The model under review builds one solid part; all positions refer to its coordinate system, in mm. Face numbers are marked on the shaded views. A direction names the side the tool comes from. Give positions to 0.01 mm unless a question says otherwise; leave off trailing zeros. Loops run counter-clockwise (first coordinate to the right, second up) from the corner with the lowest first, then second, coordinate; pieces in that order, holes last. Notation, with made-up numbers: M 8.5,-1 L 30.5,-1 A13 ccw 30.5,21 Z; hole C 18.25,31.5 d10. An arc over 180 degrees is marked long. Write item = value, one per line. Start each with the question number.
1. Draft analysis for pull direction X (two halves, no side actions). For the marked faces 1, 2, 3 and 4, state which applies: pulls with the +X half, pulls with the -X half, needs draft (parallel to the pull), parting line crosses it, or undercut.
2. We need section C-C on y = 23.5. Give the boundary of the cut face in (x, z), then the cut area to 3 significant figures.
3. For the marked faces 5 and 6, list the 3-axis set-ups (+Z, -Z, +X, -X, +Y, -Y) from which the entire face can be reached by the end or side of a thin tool; tool diameter is ignored.
4. We need section D-D on x = 61. Give the boundary of the cut face in (y, z), then the cut area to 3 significant figures.
5. We need section A-A on y = 17.5. Give the boundary of the cut face in (x, z), then the cut area to 3 significant figures.
6. We need section B-B on x = 20. Give the boundary of the cut face in (y, z).
7. For pin 1 (1.5 mm diameter, centred on x = 50.5, z = 8.5, fed in from +Y); pin 2 (4 mm diameter, centred on x = 50, z = 5, fed in from -Y); pin 3 (6 mm diameter, centred on x = 40.5, z = 7, fed in from +Y), all flat-tipped, find the tip position at first contact; note any pin that passes through.
8. Wall thickness on line 1 along X through (y, z) = (12, 1.5); line 2 along X through (y, z) = (2.55, 5); line 3 along Y through (x, z) = (17, 6): over which ranges is each line inside the solid? List them lowest first. Write a range as from..to.
from build123d import *

# Parameters (mm, degrees)
BOSS_EXTRU_1_DEPTH      = 10
CONG_1_R                = 6
ESQUISSE3_R             = 2.4
ENL_V_MAT_EXTRU_1_DEPTH = 10
ESQUISSE4_R             = 2.4
ENL_V_MAT_EXTRU_2_DEPTH = 10
ESQUISSE5_R             = 2.4
ENL_V_MAT_EXTRU_3_DEPTH = 113.249721603
CONG_2_R                = 3


with BuildPart() as part:
    # Esquisse1 → Boss.-Extru.1 (new body)
    with BuildSketch(Plane.XY):
        Polygon((25, 50), (9.188611699, 50), (24.188611699, 45), (25, 45), align=None)
        Polygon((40, 45), (25, 50), (25, 45), (30, 45), (30, 43.062870566), (40, 39.729537233), align=None)
        Polygon((25, 45), (25, 44.729537233), (30, 43.062870566), (30, 45), align=None)
        Polygon((24.188611699, 45), (25, 44.729537233), (25, 45), align=None)
        Polygon((0, 50), (0, 25), (10, 25), (10, 45), (24.188611699, 45), (9.188611699, 50), align=None)
        Polygon((0, 25), (0, 0), (25, 0), (25, 5), (10, 5), (10, 25), align=None)
        Polygon((25, 5), (25, 0), (100, 0), (100, 19.729537233), (90, 23.062870566), (90, 5), (70, 5), (70, 25), (60, 25), (60, 5), (40, 5), (40, 25), (30, 25), (30, 5), align=None)
        Polygon((30, 43.062870566), (30, 25), (40, 25), (40, 39.729537233), align=None)
        Polygon((60, 38.333333333), (40, 45), (40, 39.729537233), (60, 33.062870566), align=None)
        Polygon((70, 29.729537233), (70, 35), (60, 38.333333333), (60, 33.062870566), align=None)
        Polygon((60, 25), (70, 25), (70, 29.729537233), (60, 33.062870566), align=None)
        Polygon((84.188611699, 25), (90, 25), (90, 28.333333333), (70, 35), (70, 29.729537233), align=None)
        Polygon((90, 25), (100, 25), (90, 28.333333333), align=None)
        Polygon((90, 23.062870566), (100, 19.729537233), (100, 25), (90, 25), align=None)
        Polygon((84.188611699, 25), (90, 23.062870566), (90, 25), align=None)
    extrude(amount=BOSS_EXTRU_1_DEPTH)

    # Congé1
    cong_1_edges = [part.edges().sort_by_distance(p)[0] for p in [
        (40, 39.729537233, 5),
        (40, 5, 5),
        (60, 5, 5),
        (60, 33.062870566, 5),
        (30, 43.062870566, 5),
        (24.188611699, 45, 5),
        (10, 45, 5),
        (10, 5, 5),
        (30, 5, 5),
        (70, 29.729537233, 5),
        (70, 5, 5),
        (90, 5, 5),
        (90, 23.062870566, 5),
    ]]
    fillet(cong_1_edges, radius=CONG_1_R)

    # Esquisse3 → Enlèv. mat.-Extru.1 (cut)
    with BuildSketch(Plane(origin=(15.91886117, 47.75658351, 0), x_dir=(0.9486832980505138, -0.31622776601683805, 0), z_dir=(-0.31622776601683805, -0.9486832980505138, 0))):
        with Locations((37.924674652, 5)):
            Circle(ESQUISSE3_R)
        with Locations((69.547451254, 5)):
            Circle(ESQUISSE3_R)
    extrude(amount=-ENL_V_MAT_EXTRU_1_DEPTH, mode=Mode.SUBTRACT)

    # Esquisse4 → Enlèv. mat.-Extru.2 (cut)
    with BuildSketch(Plane.XZ):
        with Locations(Location((20, 5, 0), (0, 0, 270))):
            Circle(ESQUISSE4_R)
        with Locations(Location((50, 5, 0), (0, 0, 270))):
            Circle(ESQUISSE4_R)
        with Locations(Location((80, 5, 0), (0, 0, 270))):
            Circle(ESQUISSE4_R)
    extrude(amount=-ENL_V_MAT_EXTRU_2_DEPTH, mode=Mode.SUBTRACT)

    # Esquisse5 → Enlèv. mat.-Extru.3 (cut, through all)
    with BuildSketch(Plane(origin=(0, 50, 0), x_dir=(1, 0, 0), z_dir=(0, 1, 0))):
        with Locations(Location((20, -4.950719268, 0), (0, 0, 270))):
            Circle(ESQUISSE5_R)
    extrude(amount=-ENL_V_MAT_EXTRU_3_DEPTH, mode=Mode.SUBTRACT)

    # Congé2
    cong_2_edges = [part.edges().sort_by_distance(p)[0] for p in [
        (100, 12.5, 10),
        (0, 25, 10),
    ]]
    fillet(cong_2_edges, radius=CONG_2_R)


solid = part.part
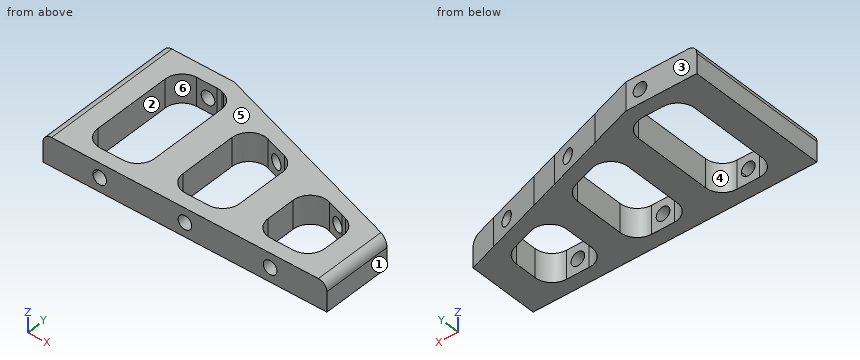
Final values:
q1.face_1 = pulls with the +X half
q1.face_2 = undercut
q1.face_3 = needs draft
q1.face_4 = undercut
q2.outline = M 0,0 L 10,0 L 10,10 L 3,10 A3 ccw 0,7 Z; M 30,0 L 40,0 L 40,10 L 30,10 Z; M 60,0 L 70.38,0 L 70.38,10 L 60,10 Z; M 87.65,0 L 100,0 L 100,7 A3 ccw 97,10 L 87.65,10 Z
q2.area = 423 mm²
q3.face_5 = +Z, +X, -X, +Y, -Y
q3.face_6 = +Z, -Z
q4.outline = M 0,0 L 38,0 L 38,10 L 0,10 Z
q4.area = 380 mm²
q5.outline = M 0,0 L 10,0 L 10,10 L 3,10 A3 ccw 0,7 Z; M 30,0 L 40,0 L 40,10 L 30,10 Z; M 60,0 L 70,0 L 70,10 L 60,10 Z; M 90,0 L 100,0 L 100,7 A3 ccw 97,10 L 90,10 Z
q5.area = 396 mm²
q6.outline = M 0,0 L 5,0 L 5,2.55 L 0,2.55 Z; M 0,7.4 L 5,7.4 L 5,10 L 0,10 Z; M 45,0 L 50,0 L 50,2.55 L 45,2.55 Z; M 45,7.35 L 50,7.35 L 50,10 L 45,10 Z
q7.pin_1 = 41.75
q7.pin_2 = 36.22
q7.pin_3 = 45.83
q8.line_1 = 0..10, 30..40, 60..70, 90..100
q8.line_2 = 0..17.6, 22.4..47.6, 52.4..77.6, 82.4..100
q8.line_3 = 0..5, 45..50
